```python
from build123d import *

# Parameters (mm, degrees)
F0_R     = 1.75
F1_DEPTH = 3
F2_R     = 4.5
F3_DEPTH = 12.5
F4_R     = 1.75
F4_R_2   = 1
F5_DEPTH = 3
F6_R     = 0.35
F7_R     = 0.45


with BuildPart() as f1:
    # F0 (on Top) → F1 (new body)
    with BuildSketch(Plane.XY):
        with BuildLine():
            Line((2, 2.5), (-2, 2.5))
            ThreePointArc((-2, 2.5), (-2.707107, 2.207107), (-3, 1.5))
            Line((-3, 1.5), (-3, -1.5))
            ThreePointArc((-3, -1.5), (-2.707107, -2.207107), (-2, -2.5))
            Line((-2, -2.5), (2, -2.5))
            ThreePointArc((2, -2.5), (2.707107, -2.207107), (3, -1.5))
            Line((3, -1.5), (3, 1.5))
            ThreePointArc((3, 1.5), (2.707107, 2.207107), (2, 2.5))
        make_face()
        Circle(F0_R, mode=Mode.SUBTRACT)
    extrude(amount=F1_DEPTH)

    # F2 (on Right) → F3 (cut, symmetric)
    with BuildSketch(Plane.YZ):
        with Locations((0, 5)):
            Circle(F2_R)
    extrude(amount=F3_DEPTH, both=True, mode=Mode.SUBTRACT)

    # F4 (on Top) → F5 (join)
    with BuildSketch(Plane.XY):
        Circle(F4_R)
        Circle(F4_R_2, mode=Mode.SUBTRACT)
    extrude(amount=F5_DEPTH)

    # F6
    f6_edges = [f1.edges().sort_by_distance(p)[0] for p in [
        (-1.75, 0, 3),
        (-1, 0, 3),
    ]]
    fillet(f6_edges, radius=F6_R)

    # F7
    f7_edges = [f1.edges().sort_by_distance(p)[0] for p in [
        (-1, 0, 0),
        (0, 2.5, 0),
        (-2.707107, 2.207107, 0),
        (-3, 0, 0),
        (-2.707107, -2.207107, 0),
        (0, -2.5, 0),
        (2.707107, -2.207107, 0),
        (3, 0, 0),
        (2.707107, 2.207107, 0),
    ]]
    fillet(f7_edges, radius=F7_R)


solid = f1.part
```
Could you check a few things on this model? Use its own coordinates, in mm. A direction names the side the tool comes from. Round coordinates to 2 decimals unless told otherwise and drop trailing zeros. Loops run counter-clockwise (first coordinate to the right, second up) from the corner with the lowest first, then second, coordinate; pieces in that order, holes last. Notation, with made-up numbers: (8, -22.5) - (28, -22.5) arc R16 ccw to (28, -11.5) - close; hole circle Ø3 at (76.5, 58.5). An arc over 180 degrees is marked (long way). Answer in a Markdown table with one row per item. Add a question column.
(1) If we section it at D-D (z = 1.9): Please give me the cut outline in (x, y).
(2) If we section it at A-A (z = 1.05): Please give me the cut outline in (x, y).
(3) I need wall thicknesses on line 1 along Y through (x, z) = (0, 1); line 2 along Y through (x, z) = (0, 1.15); line 3 along Y through (x, z) = (0, 1.5). Which ranges of each line are inside material? Lowest first, please.
(4) If we section it at B-B (y = 0): Please give me the cut outline in (x, z).
(5) If we section it at C-C (x = 0): Please give me the cut outline in (y, z), plus the area to 3 significant figures.
(6) If we mould it in two halves opening along Y, with no side actions, what happens to faces 1 (the face through (-2, 0, 0)), 2 (the face through (0, -2.5, 1)), 3 (the face through (2.6, 2.3, 0.8)), 4 (the face through (0, -1, 2))? For each: pulls with the +Y half, pulls with the -Y half, needs draft (parallel to the pull), parting line crosses it, or undercut.
(7) I'm going to push flat-ended pins straight in: pin 1 (1.6 mm diameter, centred on x = 0, y = 0, fed in from -Z); pin 2 (1.5 mm diameter, centred on y = -1, z = 2, fed in from +X). Where does each tip first touch, or does it pass through?
(8) For faces 5 (the face through (2.6, -2.3, 0.8)), 6 (the face through (0.81, -1.55, 1.56)), which set-ups out of +Z, -Z, +X, -X, +Y, -Y let a thin tool reach every point of the face, with its end or its side?
Model answer:
| question | item | result |
|---|---|---|
| 1 | outline | circle Ø3.5 at (0, 0); hole circle Ø2 at (0, 0) |
| 2 | outline | (-2.75, -2.16) arc R1 ccw to (-2, -2.5) - (2, -2.5) arc R1 ccw to (2.75, -2.16) - close; (-2.75, 2.16) - (2.75, 2.16) arc R1 ccw to (2, 2.5) - (-2, 2.5) arc R1 ccw to start; circle Ø3.5 at (0, 0); hole circle Ø2 at (0, 0) |
| 3 | line 1 | y = -2.5 to -2.06, -1.75 to -1, 1 to 1.75, 2.06 to 2.5 |
| 3 | line 2 | y = -2.5 to -2.33, -1.75 to -1, 1 to 1.75, 2.33 to 2.5 |
| 3 | line 3 | y = -1.75 to -1, 1 to 1.75 |
| 4 | outline | (-3, 0.45) arc R0.45 ccw to (-2.55, 0) - (-1.45, 0) arc R0.45 ccw to (-1, 0.45) - (-1, 2.65) arc R0.35 ccw to (-1.35, 3) - (-1.4, 3) arc R0.35 ccw to (-1.75, 2.65) - (-1.75, 0.5) - (-3, 0.5) - close; (1, 0.45) arc R0.45 ccw to (1.45, 0) - (2.55, 0) arc R0.45 ccw to (3, 0.45) - (3, 0.5) - (1.75, 0.5) - (1.75, 2.65) arc R0.35 ccw to (1.4, 3) - (1.35, 3) arc R0.35 ccw to (1, 2.65) - close |
| 5 | outline | (-2.5, 0.45) arc R0.45 ccw to (-2.05, 0) - (-1.45, 0) arc R0.45 ccw to (-1, 0.45) - (-1, 2.65) arc R0.35 ccw to (-1.35, 3) - (-1.4, 3) arc R0.35 ccw to (-1.75, 2.65) - (-1.75, 0.85) arc R4.5 cw to (-2.5, 1.26) - close; (1, 0.45) arc R0.45 ccw to (1.45, 0) - (2.05, 0) arc R0.45 ccw to (2.5, 0.45) - (2.5, 1.26) arc R4.5 cw to (1.75, 0.85) - (1.75, 2.65) arc R0.35 ccw to (1.4, 3) - (1.35, 3) arc R0.35 ccw to (1, 2.65) - close |
| 5 | area | 5.78 mm² |
| 6 | face 1 | needs draft |
| 6 | face 2 | pulls with the -Y half |
| 6 | face 3 | pulls with the +Y half |
| 6 | face 4 | undercut |
| 7 | pin 1 | passes through |
| 7 | pin 2 | stops at x = 1.73 |
| 8 | face 5 | +Z, -Z, +X, -Y |
| 8 | face 6 | +Z |
